Study the drawing (mm; zero at the part's minimum x, y, z) and answer. A direction names the side the tool comes from. Give positions to 0.01 mm unless a question says otherwise; leave off trailing zeros. Write each loop counter-clockwise with the first axis right and the second up, starting at its lowest first coordinate (ties: lowest second). Pieces come first, ordered by that corner, then holes.
1) Determine the mould class of the marked faces 4, 5 and 6 for opening direction Z: pulls with the +Z half, pulls with the -Z half, needs draft (parallel to the pull), parting line crosses it, or undercut.
2) Given pin 1 Ø7 at (y, z) = (50, 8) entering from +X; pin 2 Ø1.8 at (x, z) = (12, 9.5) entering from -Y; pin 3 Ø4.5 at (x, z) = (13, 5) entering from +Y; pin 4 Ø7 at (x, y) = (12.5, 7) entering from +Z, each flat-ended and moving along its own axis, determine where each tip first touches the part or whether it passes through.
3) Straight lines are drawn through the part: probe 1 along Y at (x, z) = (12.5, 13.45); probe 2 along Z at (x, y) = (19, 33); probe 3 along X at (y, z) = (54, 12). For each, find the intervals that lie inside material, in ascending order.
4) Find section C-C (x = 12.5). Determine the outline of the cut face in (y, z), plus the area to 3 significant figures.
5) Find section A-A (y = 7). Determine the outline of the cut face in (x, z).
6) A tool of negligible diameter and unlimited length cuts with its end or side. For the marked faces 1, 2 and 3, from which of +Z, -Z, +X, -X, +Y, -Y can it reach the whole face along a straight path? Write none if from no direction.
7) Find section B-B (y = 46). Determine the outline of the cut face in (x, z), plus the area to 3 significant figures.
8) Find section D-D (z = 1). Determine the outline of the cut face in (x, y).
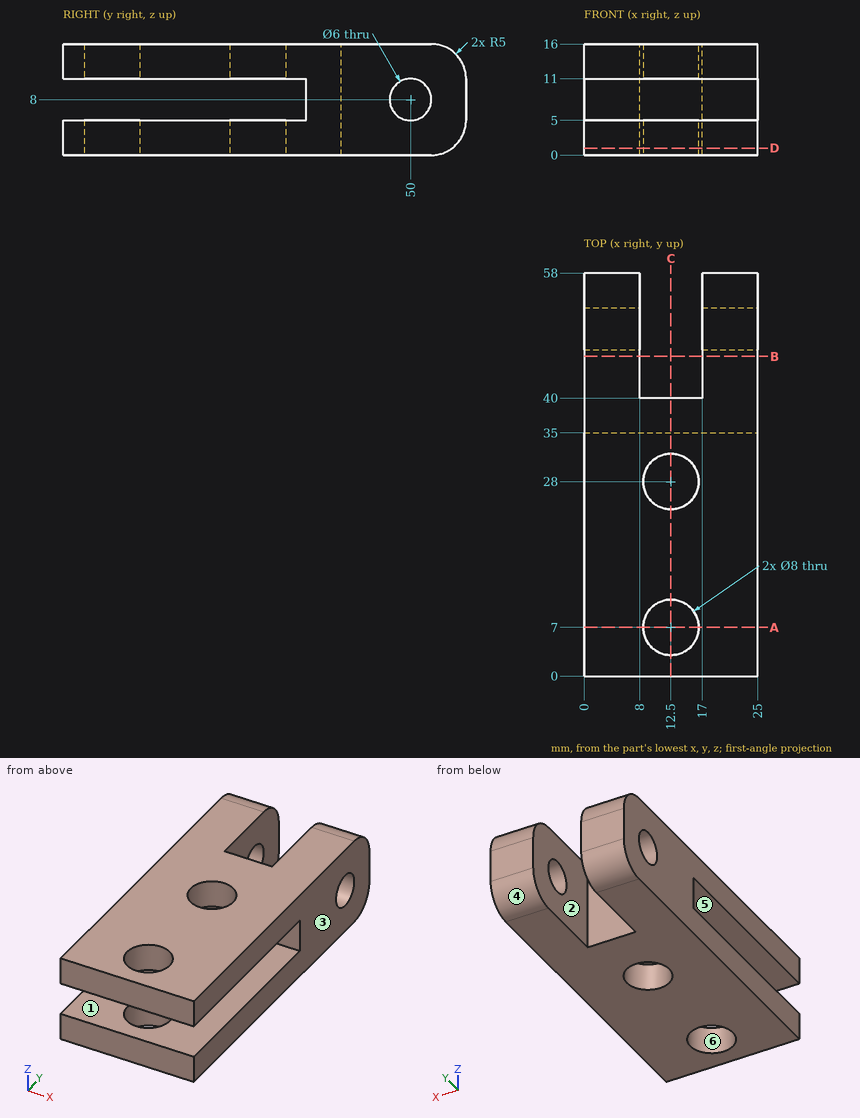
Results:
1. face 4: pulls with the -Z half
1. face 5: undercut
1. face 6: needs draft
2. pin 1: stops at x = 25
2. pin 2: stops at y = 35
2. pin 3: stops at y = 40
2. pin 4: passes through
3. probe 1: y = 0 to 3, 11 to 24, 32 to 40
3. probe 2: z = 0 to 5, 11 to 16
3. probe 3: x = 0 to 8, 17 to 25
4. outline: (0, 0) - (3, 0) - (3, 5) - (0, 5) - close; (0, 11) - (3, 11) - (3, 16) - (0, 16) - close; (11, 0) - (24, 0) - (24, 5) - (11, 5) - close; (11, 11) - (24, 11) - (24, 16) - (11, 16) - close; (32, 0) - (40, 0) - (40, 16) - (32, 16) - (32, 11) - (35, 11) - (35, 5) - (32, 5) - close
4. area: 270 mm2
5. outline: (0, 0) - (8.5, 0) - (8.5, 5) - (0, 5) - close; (0, 11) - (8.5, 11) - (8.5, 16) - (0, 16) - close; (16.5, 0) - (25, 0) - (25, 5) - (16.5, 5) - close; (16.5, 11) - (25, 11) - (25, 16) - (16.5, 16) - close
6. face 1: +X, -X, -Y
6. face 2: +Z, -Z, +Y
6. face 3: +Z, -Z, +X, +Y, -Y
7. outline: (0, 0) - (8, 0) - (8, 16) - (0, 16) - close; (17, 0) - (25, 0) - (25, 16) - (17, 16) - close
7. area: 256 mm2
8. outline: (0, 0) - (25, 0) - (25, 56) - (17, 56) - (17, 40) - (8, 40) - (8, 56) - (0, 56) - close; hole circle Ø8 at (12.5, 7); hole circle Ø8 at (12.5, 28)
